For this review, use the dimensioned drawing (mm, ordinates from the lowest corner) and the shaded views. Round coordinates to 2 decimals unless told otherwise and drop trailing zeros. Write each loop counter-clockwise with the first axis right and the second up, starting at its lowest first coordinate (ties: lowest second). Pieces come first, ordered by that corner, then holes.
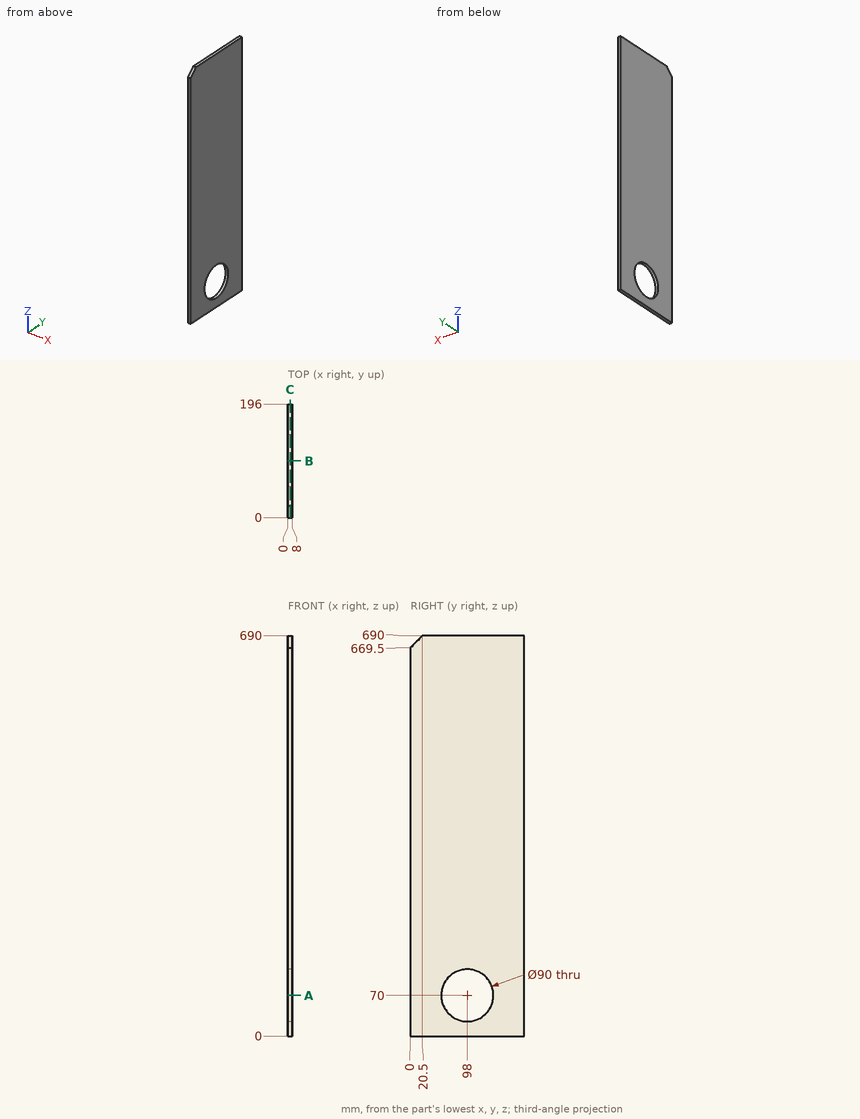
(1) For line 1 along Y through (x, z) = (3.75, 70); line 2 along Z through (x, y) = (7, 75.5); line 3 along Z through (x, y) = (6.5, 63.5), list the stretches that pass through material, from the lowest coordinate up.
Geometry check:
line 1: y = 0 to 53, 143 to 196
line 2: z = 0 to 31.03, 108.97 to 690
line 3: z = 0 to 41.11, 98.89 to 690
(2) We need section B-B, the plane y = 98. Give the boundary of the cut face in (x, z).
Geometry check:
outline: (0, 0) - (8, 0) - (8, 25) - (0, 25) - close; (0, 115) - (8, 115) - (8, 690) - (0, 690) - close
(3) We need section A-A, the plane z = 70. Give the boundary of the cut face in (x, y), and give its area (3 significant figures).
Geometry check:
outline: (0, 0) - (8, 0) - (8, 53) - (0, 53) - close; (0, 143) - (8, 143) - (8, 196) - (0, 196) - close
area: 848 mm2
(4) We need section C-C, the plane x = 3.75. Give the boundary of the cut face in (y, z).
Geometry check:
outline: (0, 0) - (196, 0) - (196, 690) - (20.5, 690) - (0, 669.5) - close; hole circle Ø90 at (98, 70)
